```python
from build123d import *

# Parameters (mm, degrees)
SKETCH3_W           = 228.6
SKETCH3_H           = 266.7
SKETCH3_R           = 2.54
SKETCH3_W_2         = 193.04
SKETCH3_H_2         = 82.55
BOSS_EXTRUDE3_DEPTH = 2.286
FILLET5_R           = 12.7
FILLET6_R           = 6.35


with BuildPart() as part:
    # Sketch3 → Boss-Extrude3 (new body)
    with BuildSketch(Plane(origin=(0, 0, 0), x_dir=(1, 0, 0), z_dir=(0, 1, 0))):
        with Locations((114.3, 133.35)):
            Rectangle(SKETCH3_W, SKETCH3_H)
        with Locations(Location((12.7, 254, 0), (0, 0, 270))):
            Circle(SKETCH3_R, mode=Mode.SUBTRACT)
        with Locations(Location((25.4, 254, 0), (0, 0, 270))):
            Circle(SKETCH3_R, mode=Mode.SUBTRACT)
        with Locations(Location((38.1, 254, 0), (0, 0, 270))):
            Circle(SKETCH3_R, mode=Mode.SUBTRACT)
        with Locations(Location((50.8, 254, 0), (0, 0, 270))):
            Circle(SKETCH3_R, mode=Mode.SUBTRACT)
        with Locations(Location((63.5, 254, 0), (0, 0, 270))):
            Circle(SKETCH3_R, mode=Mode.SUBTRACT)
        with Locations(Location((76.2, 254, 0), (0, 0, 270))):
            Circle(SKETCH3_R, mode=Mode.SUBTRACT)
        with Locations(Location((88.9, 254, 0), (0, 0, 270))):
            Circle(SKETCH3_R, mode=Mode.SUBTRACT)
        with Locations(Location((101.6, 254, 0), (0, 0, 270))):
            Circle(SKETCH3_R, mode=Mode.SUBTRACT)
        with Locations(Location((114.3, 254, 0), (0, 0, 270))):
            Circle(SKETCH3_R, mode=Mode.SUBTRACT)
        with Locations(Location((127, 254, 0), (0, 0, 270))):
            Circle(SKETCH3_R, mode=Mode.SUBTRACT)
        with Locations(Location((139.7, 254, 0), (0, 0, 270))):
            Circle(SKETCH3_R, mode=Mode.SUBTRACT)
        with Locations(Location((152.4, 254, 0), (0, 0, 270))):
            Circle(SKETCH3_R, mode=Mode.SUBTRACT)
        with Locations(Location((165.1, 254, 0), (0, 0, 270))):
            Circle(SKETCH3_R, mode=Mode.SUBTRACT)
        with Locations(Location((177.8, 254, 0), (0, 0, 270))):
            Circle(SKETCH3_R, mode=Mode.SUBTRACT)
        with Locations(Location((190.5, 254, 0), (0, 0, 270))):
            Circle(SKETCH3_R, mode=Mode.SUBTRACT)
        with Locations(Location((203.2, 254, 0), (0, 0, 270))):
            Circle(SKETCH3_R, mode=Mode.SUBTRACT)
        with Locations(Location((215.9, 254, 0), (0, 0, 270))):
            Circle(SKETCH3_R, mode=Mode.SUBTRACT)
        with Locations(Location((25.4, 241.3, 0), (0, 0, 270))):
            Circle(SKETCH3_R, mode=Mode.SUBTRACT)
        with Locations(Location((38.1, 241.3, 0), (0, 0, 270))):
            Circle(SKETCH3_R, mode=Mode.SUBTRACT)
        with Locations(Location((50.8, 241.3, 0), (0, 0, 270))):
            Circle(SKETCH3_R, mode=Mode.SUBTRACT)
        with Locations(Location((63.5, 241.3, 0), (0, 0, 270))):
            Circle(SKETCH3_R, mode=Mode.SUBTRACT)
        with Locations(Location((76.2, 241.3, 0), (0, 0, 270))):
            Circle(SKETCH3_R, mode=Mode.SUBTRACT)
        with Locations(Location((88.9, 241.3, 0), (0, 0, 270))):
            Circle(SKETCH3_R, mode=Mode.SUBTRACT)
        with Locations(Location((101.6, 241.3, 0), (0, 0, 270))):
            Circle(SKETCH3_R, mode=Mode.SUBTRACT)
        with Locations(Location((114.3, 241.3, 0), (0, 0, 270))):
            Circle(SKETCH3_R, mode=Mode.SUBTRACT)
        with Locations(Location((127, 241.3, 0), (0, 0, 270))):
            Circle(SKETCH3_R, mode=Mode.SUBTRACT)
        with Locations(Location((139.7, 241.3, 0), (0, 0, 270))):
            Circle(SKETCH3_R, mode=Mode.SUBTRACT)
        with Locations(Location((152.4, 241.3, 0), (0, 0, 270))):
            Circle(SKETCH3_R, mode=Mode.SUBTRACT)
        with Locations(Location((165.1, 241.3, 0), (0, 0, 270))):
            Circle(SKETCH3_R, mode=Mode.SUBTRACT)
        with Locations(Location((177.8, 241.3, 0), (0, 0, 270))):
            Circle(SKETCH3_R, mode=Mode.SUBTRACT)
        with Locations(Location((190.5, 241.3, 0), (0, 0, 270))):
            Circle(SKETCH3_R, mode=Mode.SUBTRACT)
        with Locations(Location((203.2, 241.3, 0), (0, 0, 270))):
            Circle(SKETCH3_R, mode=Mode.SUBTRACT)
        with Locations(Location((215.9, 241.3, 0), (0, 0, 270))):
            Circle(SKETCH3_R, mode=Mode.SUBTRACT)
        with Locations(Location((25.4, 228.6, 0), (0, 0, 270))):
            Circle(SKETCH3_R, mode=Mode.SUBTRACT)
        with Locations(Location((38.1, 228.6, 0), (0, 0, 270))):
            Circle(SKETCH3_R, mode=Mode.SUBTRACT)
        with Locations(Location((50.8, 228.6, 0), (0, 0, 270))):
            Circle(SKETCH3_R, mode=Mode.SUBTRACT)
        with Locations(Location((63.5, 228.6, 0), (0, 0, 270))):
            Circle(SKETCH3_R, mode=Mode.SUBTRACT)
        with Locations(Location((76.2, 228.6, 0), (0, 0, 270))):
            Circle(SKETCH3_R, mode=Mode.SUBTRACT)
        with Locations(Location((88.9, 228.6, 0), (0, 0, 270))):
            Circle(SKETCH3_R, mode=Mode.SUBTRACT)
        with Locations(Location((101.6, 228.6, 0), (0, 0, 270))):
            Circle(SKETCH3_R, mode=Mode.SUBTRACT)
        with Locations(Location((114.3, 228.6, 0), (0, 0, 270))):
            Circle(SKETCH3_R, mode=Mode.SUBTRACT)
        with Locations(Location((127, 228.6, 0), (0, 0, 270))):
            Circle(SKETCH3_R, mode=Mode.SUBTRACT)
        with Locations(Location((139.7, 228.6, 0), (0, 0, 270))):
            Circle(SKETCH3_R, mode=Mode.SUBTRACT)
        with Locations(Location((152.4, 228.6, 0), (0, 0, 270))):
            Circle(SKETCH3_R, mode=Mode.SUBTRACT)
        with Locations(Location((165.1, 228.6, 0), (0, 0, 270))):
            Circle(SKETCH3_R, mode=Mode.SUBTRACT)
        with Locations(Location((177.8, 228.6, 0), (0, 0, 270))):
            Circle(SKETCH3_R, mode=Mode.SUBTRACT)
        with Locations(Location((190.5, 228.6, 0), (0, 0, 270))):
            Circle(SKETCH3_R, mode=Mode.SUBTRACT)
        with Locations(Location((203.2, 228.6, 0), (0, 0, 270))):
            Circle(SKETCH3_R, mode=Mode.SUBTRACT)
        with Locations(Location((215.9, 228.6, 0), (0, 0, 270))):
            Circle(SKETCH3_R, mode=Mode.SUBTRACT)
        with Locations(Location((12.7, 241.3, 0), (0, 0, 270))):
            Circle(SKETCH3_R, mode=Mode.SUBTRACT)
        with Locations(Location((12.7, 228.6, 0), (0, 0, 270))):
            Circle(SKETCH3_R, mode=Mode.SUBTRACT)
        with Locations(Location((12.7, 12.7, 0), (0, 0, 270))):
            Circle(SKETCH3_R, mode=Mode.SUBTRACT)
        with Locations(Location((25.4, 12.7, 0), (0, 0, 270))):
            Circle(SKETCH3_R, mode=Mode.SUBTRACT)
        with Locations(Location((38.1, 12.7, 0), (0, 0, 270))):
            Circle(SKETCH3_R, mode=Mode.SUBTRACT)
        with Locations(Location((50.8, 12.7, 0), (0, 0, 270))):
            Circle(SKETCH3_R, mode=Mode.SUBTRACT)
        with Locations(Location((63.5, 12.7, 0), (0, 0, 270))):
            Circle(SKETCH3_R, mode=Mode.SUBTRACT)
        with Locations(Location((76.2, 12.7, 0), (0, 0, 270))):
            Circle(SKETCH3_R, mode=Mode.SUBTRACT)
        with Locations(Location((88.9, 12.7, 0), (0, 0, 270))):
            Circle(SKETCH3_R, mode=Mode.SUBTRACT)
        with Locations(Location((101.6, 12.7, 0), (0, 0, 270))):
            Circle(SKETCH3_R, mode=Mode.SUBTRACT)
        with Locations(Location((114.3, 12.7, 0), (0, 0, 270))):
            Circle(SKETCH3_R, mode=Mode.SUBTRACT)
        with Locations(Location((127, 12.7, 0), (0, 0, 270))):
            Circle(SKETCH3_R, mode=Mode.SUBTRACT)
        with Locations(Location((139.7, 12.7, 0), (0, 0, 270))):
            Circle(SKETCH3_R, mode=Mode.SUBTRACT)
        with Locations(Location((152.4, 12.7, 0), (0, 0, 270))):
            Circle(SKETCH3_R, mode=Mode.SUBTRACT)
        with Locations(Location((165.1, 12.7, 0), (0, 0, 270))):
            Circle(SKETCH3_R, mode=Mode.SUBTRACT)
        with Locations(Location((177.8, 12.7, 0), (0, 0, 270))):
            Circle(SKETCH3_R, mode=Mode.SUBTRACT)
        with Locations(Location((190.5, 12.7, 0), (0, 0, 270))):
            Circle(SKETCH3_R, mode=Mode.SUBTRACT)
        with Locations(Location((203.2, 12.7, 0), (0, 0, 270))):
            Circle(SKETCH3_R, mode=Mode.SUBTRACT)
        with Locations(Location((215.9, 12.7, 0), (0, 0, 270))):
            Circle(SKETCH3_R, mode=Mode.SUBTRACT)
        with Locations(Location((12.7, 114.3, 0), (0, 0, 270))):
            Circle(SKETCH3_R, mode=Mode.SUBTRACT)
        with Locations(Location((63.5, 114.3, 0), (0, 0, 270))):
            Circle(SKETCH3_R, mode=Mode.SUBTRACT)
        with Locations(Location((114.3, 114.3, 0), (0, 0, 270))):
            Circle(SKETCH3_R, mode=Mode.SUBTRACT)
        with Locations(Location((165.1, 114.3, 0), (0, 0, 270))):
            Circle(SKETCH3_R, mode=Mode.SUBTRACT)
        with Locations(Location((215.9, 114.3, 0), (0, 0, 270))):
            Circle(SKETCH3_R, mode=Mode.SUBTRACT)
        with Locations(Location((12.7, 165.1, 0), (0, 0, 270))):
            Circle(SKETCH3_R, mode=Mode.SUBTRACT)
        with Locations(Location((215.9, 165.1, 0), (0, 0, 270))):
            Circle(SKETCH3_R, mode=Mode.SUBTRACT)
        with Locations(Location((12.7, 63.5, 0), (0, 0, 270))):
            Circle(SKETCH3_R, mode=Mode.SUBTRACT)
        with Locations(Location((215.9, 63.5, 0), (0, 0, 270))):
            Circle(SKETCH3_R, mode=Mode.SUBTRACT)
        with Locations((114.3, 66.675)):
            Rectangle(SKETCH3_W_2, SKETCH3_H_2, mode=Mode.SUBTRACT)
        with Locations((114.3, 168.275)):
            Rectangle(SKETCH3_W_2, SKETCH3_H_2, mode=Mode.SUBTRACT)
    extrude(amount=BOSS_EXTRUDE3_DEPTH)

    # Fillet5
    fillet5_edges = [part.edges().sort_by_distance(p)[0] for p in [
        (0, 1.143, -266.7),
        (228.6, 1.143, -266.7),
        (228.6, 1.143, 0),
        (0, 1.143, 0),
    ]]
    fillet(fillet5_edges, radius=FILLET5_R)

    # Fillet6
    fillet6_edges = [part.edges().sort_by_distance(p)[0] for p in [
        (210.82, 1.143, -107.95),
        (17.78, 1.143, -107.95),
        (17.78, 1.143, -25.4),
        (210.82, 1.143, -25.4),
        (17.78, 1.143, -209.55),
        (17.78, 1.143, -127),
        (210.82, 1.143, -127),
        (210.82, 1.143, -209.55),
    ]]
    fillet(fillet6_edges, radius=FILLET6_R)


solid = part.part
```
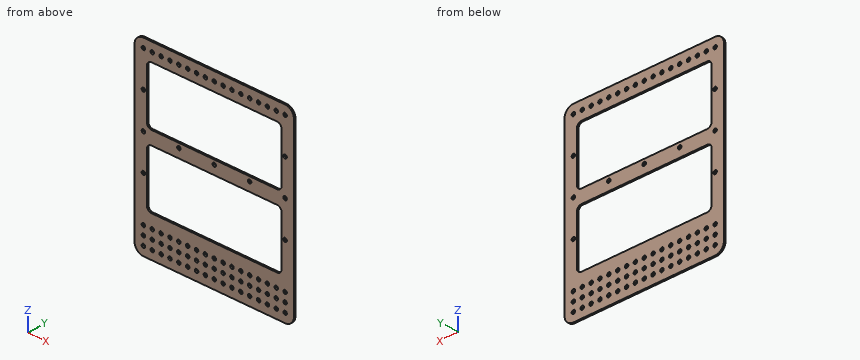
Geometry check sheet. Reference: the model listing, model coordinates, mm. Give positions to 0.01 mm unless a question says otherwise; leave off trailing zeros. Order: outer loops, then holes, each group sorted by start corner. A loop starts at its lowest first (then second) coordinate and runs counter-clockwise, first axis right, second up. Notation, with made-up numbers: (9.25, 24.25) - (56.25, 24.25) arc R26 ccw to (56.25, 44.25) - close; hole circle Ø10 at (47, 7.5). An arc over 180 degrees is marked (long way). Answer in a Markdown table with one row per item. Add a question column.
Q1. Cross-section at B-B, the plane x = 32. Enter the section's corners in (y, z).
Q2. Material ranges on probe 1 along Z at (x, y) = (59, 1.7); probe 2 along X at (y, z) = (1.45, -92); probe 3 along X at (y, z) = (1.05, -114.5), recorded low to high. Write a range as from..to.
Q3. Cross-section at C-C, the plane y = 1. Count the separate pieces of the cut face and the enclosed holes in it, then the cut area to 3 significant figures.
Q4. Gauge pin test, flat end, axial feed: pin 1 (3 mm diameter, centred on x = 190.5, z = -228.6, fed in from -Y). Record the tip position at first contact, or that the pin passes through.
Q5. Cross-section at A-A, the plane z = -98.5. Enter the section's corners in (x, y), then the cut area to 3 significant figures.
Check values:
| question | item | result |
|---|---|---|
| 1 | outline | (0, -266.7) - (2.29, -266.7) - (2.29, -209.55) - (0, -209.55) - close; (0, -127) - (2.29, -127) - (2.29, -107.95) - (0, -107.95) - close; (0, -25.4) - (2.29, -25.4) - (2.29, 0) - (0, 0) - close |
| 2 | probe 1 | z = -266.7..-209.55, -127..-107.95, -25.4..0 |
| 2 | probe 2 | x = 0..17.78, 210.82..228.6 |
| 2 | probe 3 | x = 0..10.17, 15.23..60.97, 66.03..111.77, 116.83..162.57, 167.63..213.37, 218.43..228.6 |
| 3 | separate pieces | 1 |
| 3 | enclosed holes | 79 |
| 3 | area | 27,500 mm^2 |
| 4 | pin 1 | passes through |
| 5 | outline | (0, 0) - (17.78, 0) - (17.78, 2.29) - (0, 2.29) - close; (210.82, 0) - (228.6, 0) - (228.6, 2.29) - (210.82, 2.29) - close |
| 5 | area | 81.3 mm^2 |
